Drawing for the job (mm, zero at the part's lowest x, y, z). A direction names the side the tool comes from. Coordinates: 2 decimals unless noted, no trailing zeros. Write each loop counter-clockwise with the first axis right and the second up, starting at its lowest first coordinate (ties: lowest second). Pieces come first, ordered by that corner, then holes. Notation, with made-up numbers: (-16.5, 13.5) -> (34.5, 13.5) arc R27 ccw to (34.5, 33.5) -> close; hole circle Ø7 at (52.5, 59.5). An arc over 180 degrees is marked (long way). Write item = value, one per line. Start each with the question number.
Q1. Band-saw the part on B-B, the plane y = 7.5. Give the number of separate pieces and of enclosed holes in the cut face, plus the area to 3 significant figures.
Q2. Pin check, flat tips, straight feed: P1, Ø3, axis at x = 18, y = 4, coming from the -Z side; P2, Ø7.5, axis at y = 7.5, z = 25, coming from the +X side; P3, Ø2.5, axis at x = 16, y = 6.5, coming from the +Z side. Stop position of each tip, or through.
Q3. Band-saw the part on C-C, the plane z = 18.5. List the corners of the cut face in (x, y).
Q4. Probe line 1 (X direction, y = 11, z = 28); line 2 (X direction, y = 5.5, z = 21); line 3 (Y direction, x = 19.15, z = 25). List the from-to ranges inside material, lowest first.
Q5. Tool access for the marked faces 5, 6, 7 and 8: list every direction of +Z, -Z, +X, -X, +Y, -Y with a clear straight run to the whole face (end or side of a thin tool).
Q6. Band-saw the part on D-D, the plane x = 18.25. List the corners of the cut face in (y, z).
Q7. Band-saw the part on A-A, the plane z = 3.5. List the corners of the cut face in (x, y).
Q8. Pull direction Z, two halves, no side cores. Call the marked faces 1, 2, 3 and 4: released by +Z, released by -Z, zero draft, split by the parting line, or undercut.
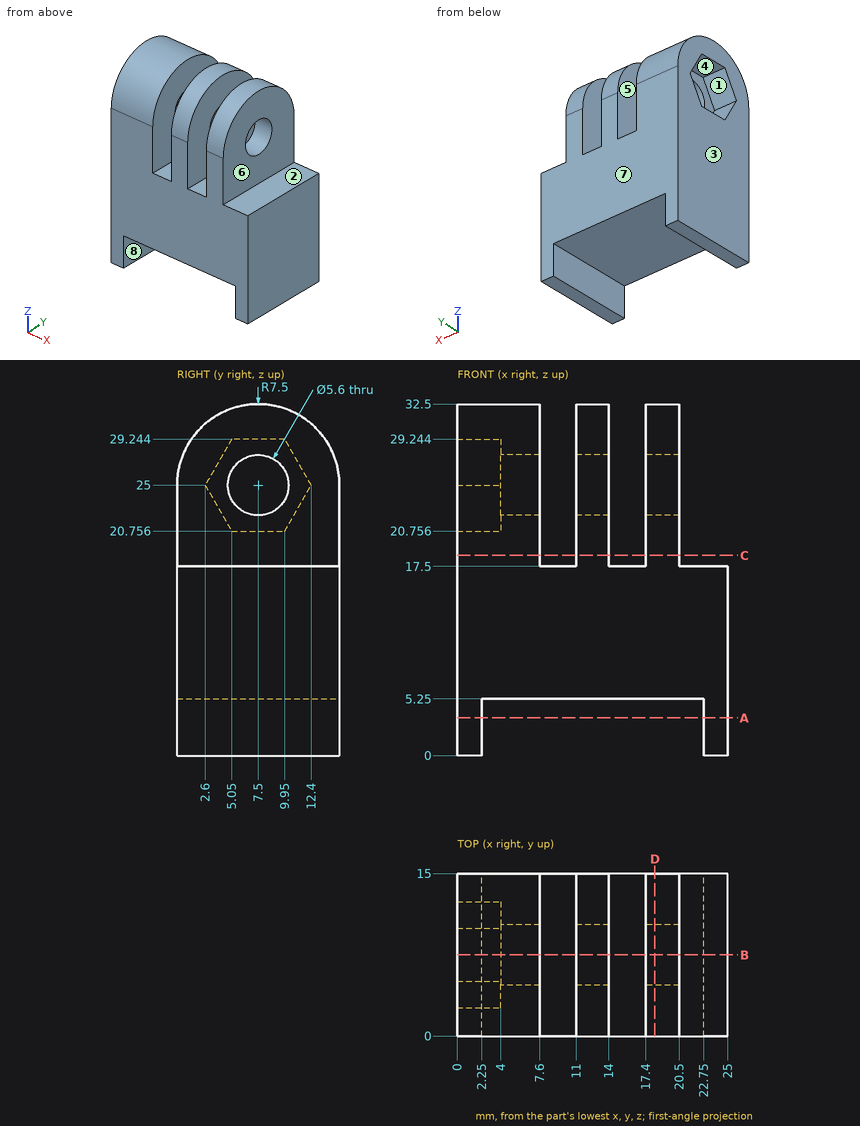
Ans:
q1.separate_pieces = 4
q1.enclosed_holes = 0
q1.area = 447 mm2
q2.P1 = 5.25
q2.P2 = 20.5
q2.P3 = 17.5
q3.outline = (0, 0) -> (7.6, 0) -> (7.6, 15) -> (0, 15) -> close; (11, 0) -> (14, 0) -> (14, 15) -> (11, 15) -> close; (17.4, 0) -> (20.5, 0) -> (20.5, 15) -> (17.4, 15) -> close
q4.line_1 = 0 to 7.6, 11 to 14, 17.4 to 20.5
q4.line_2 = 4 to 7.6, 11 to 14, 17.4 to 20.5
q4.line_3 = 0 to 4.7, 10.3 to 15
q5.face_5 = +Z, +Y, -Y
q5.face_6 = +Z, +X, +Y, -Y
q5.face_7 = +Z, -Z, +X, -X, +Y
q5.face_8 = -Z, +Y, -Y
q6.outline = (0, 5.25) -> (15, 5.25) -> (15, 25) arc R7.5 ccw to (0, 25) -> close; hole circle Ø5.6 at (7.5, 25)
q7.outline = (0, 0) -> (2.25, 0) -> (2.25, 15) -> (0, 15) -> close; (22.75, 0) -> (25, 0) -> (25, 15) -> (22.75, 15) -> close
q8.face_1 = undercut
q8.face_2 = released by +Z
q8.face_3 = zero draft
q8.face_4 = undercut
